Autodesk Inventor part; units mm, degrees
ref_plane "YZ Plane" through (0, 0, 0) normal (1, 0, 0) x (0, 1, 0)
ref_plane "XZ Plane" through (0, 0, 0) normal (0, 1, 0) x (-1, 0, 0)
ref_plane "XY Plane" through (0, 0, 0) normal (0, 0, 1) x (1, 0, 0)
sketch "Sketch1" plane through (0, 0, 0) normal (0, 1, 0) x (-1, 0, 0)
  circle A0 centre (0, 0) radius 2.3241
  line L0 (0, 0) -> (0, -38.1)
  circle A1 centre (0, -38.1) radius 2.3241
  line L1 (0, 0) -> (0, -38.1) construction
  line L2 (-6.35, 0) -> (-6.35, -38.1)
  line L3 (6.35, -38.1) -> (6.35, 0)
  arc A2 (6.35, 0) -> (-6.35, 0) centre (0, 0) ccw
  arc A3 (-6.35, -38.1) -> (6.35, -38.1) centre (0, -38.1) ccw
  line L4 (0, -38.1) -> (-15.9411, -38.1) construction
  line L5 (0, -31.75) -> (-15.9411, -31.75)
  line L6 (-15.9411, -44.45) -> (0, -44.45)
  arc A4 (0, -44.45) -> (0, -31.75) centre (0, -38.1) ccw
  arc A5 (-15.9411, -31.75) -> (-15.9411, -44.45) centre (-15.9411, -38.1) ccw
  line L7 (-5.9094, 2.3241) -> (-21.799, -35.6488)
  point P0 (0, -19.05)
  point P1 (-7.9706, -38.1)
  dimension "d0" = 4.6482
  dimension "d1" = 38.1
  dimension "d2" = 4.6482
  dimension "d3" = 12.7
extrude "Extrusion1" add sketch "Sketch1" along normal blind 1.5875
sketch "Sketch2" plane through (0, 1.5875, 0) normal (0, 1, 0) x (1, 0, 0)
  circle A0 centre (0, 38.1) radius 2.3241
  line L0 (0, 38.1) -> (0, 31.75)
  line L1 (0, 31.75) -> (0, 92.71) construction
  line L2 (6.35, 38.1) -> (6.35, 86.36)
  line L3 (-6.35, 86.36) -> (-6.35, 38.1)
  arc A1 (-6.35, 38.1) -> (6.35, 38.1) centre (0, 38.1) ccw
  arc A2 (6.35, 86.36) -> (-6.35, 86.36) centre (0, 86.36) ccw
  line L4 (-6.35, 86.36) -> (57.15, 86.36) construction
  line L5 (0, 80.01) -> (50.8, 80.01)
  line L6 (50.8, 92.71) -> (0, 92.71)
  arc A3 (0, 92.71) -> (0, 80.01) centre (0, 86.36) ccw
  arc A4 (50.8, 80.01) -> (50.8, 92.71) centre (50.8, 86.36) ccw
  line L7 (-6.35, 38.1) -> (-6.35, 0)
  arc A5 (-6.35, 0) -> (5.9094, -2.3241) centre (0, 0) ccw
  line L8 (5.9094, -2.3241) -> (21.799, 35.6488)
  arc A6 (21.799, 35.6488) -> (15.9411, 44.45) centre (15.9411, 38.1) ccw
  line L9 (15.9411, 44.45) -> (0, 44.45)
  arc A7 (0, 44.45) -> (-6.35, 38.1) centre (0, 38.1) ccw
  circle A8 centre (0, 0) radius 2.3241
  circle A9 centre (0, 38.1) radius 2.3241
  line L10 (21.799, 35.6488) -> (55.9369, 82.6271)
  point P0 (0, 62.23)
  point P1 (25.4, 86.36)
  point P2 (0, 92.71)
  point P3 (6.35, 44.45)
  dimension "d6" = 6.35
  dimension "d7" = 60.96
  dimension "d10" = 63.5
extrude "Extrusion2" add sketch "Sketch2" against normal blind 1.5875 contours A1 A7 L9 L2 | L9 A7 L3 A3 L5 L2 | L2 L5 A4 L10 A6 L9 | L5 A3 A2 L2 | L2 A2 L6 A4 L5
sketch "Sketch3" plane through (0, 1.5875, 0) normal (0, 1, 0) x (1, 0, 0)
  arc A0 (55.9369, 82.6271) -> (50.8, 92.71) centre (50.8, 86.36) ccw
  line L0 (5.9094, -2.3241) -> (21.799, 35.6488)
  arc A1 (55.9369, 82.6271) -> (5.9094, -2.3241) centre (174.4039, -44.3439) ccw
  line L1 (21.799, 35.6488) -> (55.9369, 82.6271)
  point P0 (0, 0)
extrude "Extrusion3" cut sketch "Sketch3" against normal blind 1.5875
sketch "Sketch4" plane through (0, 1.5875, 0) normal (0, 1, 0) x (1, 0, 0)
  line L0 (0, 92.71) -> (50.8, 92.71)
  line L1 (-6.35, 86.36) -> (-6.35, 0)
  arc A0 (30.6634, 92.71) -> (-6.35, 43.18) centre (81.4918, 16.1314) ccw
  arc A1 (55.9369, 82.6271) -> (5.9094, -2.3241) centre (174.4039, -44.3439) ccw
  arc A2 (55.9369, 82.6271) -> (50.8, 92.71) centre (50.8, 86.36) ccw
  line L2 (50.8, 92.71) -> (0, 92.71)
  arc A3 (0, 92.71) -> (-6.35, 86.36) centre (0, 86.36) ccw
  line L3 (-6.35, 86.36) -> (-6.35, 0)
  arc A4 (-6.35, 0) -> (5.9094, -2.3241) centre (0, 0) ccw
  circle A5 centre (0, 0) radius 2.3241
  circle A6 centre (0, 38.1) radius 2.3241
extrude "Extrusion4" cut sketch "Sketch4" against normal blind 1.5875 contours L0 A0 L1 A3
sketch "Sketch5" plane through (0, 1.5875, 0) normal (0, 1, 0) x (1, 0, 0)
  point P0 (0, 0)
sketch "Sketch6" plane through (0, 1.5875, 0) normal (0, 1, 0) x (1, 0, 0)
  circle A0 centre (0, 38.1) radius 2.3241
  line L0 (0, 38.1) -> (0, 50.8)
  circle A1 centre (0, 50.8) radius 2.3241
  point P0 (0, 0)
  dimension "d15" = 12.7
  dimension "d16" = 4.6482
extrude "Extrusion5" cut sketch "Sketch6" against normal blind 1.5875 contours A1
sketch "Sketch7" plane through (0, 1.5875, 0) normal (0, 1, 0) x (1, 0, 0)
  circle A0 centre (0, 50.8) radius 2.3241
  circle A1 centre (0, 38.1) radius 2.3241
  arc A2 (6.2992, 38.1) -> (-6.2992, 38.1) centre (0, 38.1) ccw
  circle A3 centre (0, 38.1) radius 2.3241
  line L0 (0, 50.8) -> (0, 88.9)
  arc A4 (35.4436, 84.1127) -> (5.3749, 48.0302) centre (101.5031, -1.5067) ccw
  arc A5 (31.75, 88.9) -> (0, 50.8) centre (101.5031, -1.5067) ccw
  arc A6 (31.75, 88.9) -> (0, 50.8) centre (101.5031, -1.5067) ccw construction
  arc A7 (28.0564, 93.6873) -> (-5.3749, 53.5698) centre (101.5031, -1.5067) ccw
  line L1 (0, 88.9) -> (31.75, 88.9)
  arc A8 (35.4436, 84.1127) -> (28.0564, 93.6873) centre (31.75, 88.9) ccw
  line L2 (0, 50.8) -> (6.2992, 50.8)
  circle A9 centre (0, 50.8) radius 2.3241
  arc A10 (6.2992, 50.8) -> (-6.2992, 50.8) centre (0, 50.8) ccw
  line L3 (-6.2992, 50.8) -> (0, 50.8)
  arc A11 (-5.3749, 53.5698) -> (5.3749, 48.0302) centre (0, 50.8) ccw
  line L4 (-6.2992, 38.1) -> (-6.2992, 50.8)
  line L5 (0, 38.1) -> (0, 50.8) construction
  line L6 (6.2992, 50.8) -> (6.2992, 38.1)
  circle A12 centre (0, 38.1) radius 2.3241
  circle A13 centre (31.75, 88.9) radius 2.3241
  point P0 (0, 0)
  point P1 (0, 44.45)
  point P2 (-4.5326, 55.1744)
  point P3 (6.2992, 49.7843)
  point P4 (0, 57.0992)
  point P5 (2.3241, 50.8)
  point P6 (0, 53.1241)
  dimension "d19" = 4.6482
  dimension "d40" = 4.6482
extrude "Extrusion6" add sketch "Sketch7" against normal blind 1.5875 contours L2 L6 A4 A11 L3 A0 | L3 A11 A7 A10 L0 A0 | A10 A5 A13 L1 A7 A8 A4 L6 | A10 L0 A7 L1 A13 A5 | A11 A4 L6 A2 L4 L3 | L3 A10 A7 A11 | A10 A7 L0 | A13 L1 A5 | A5 L1 A13
sketch "Sketch8" plane through (0, 1.5875, 0) normal (0, 1, 0) x (1, 0, 0)
  circle A0 centre (0, 50.8) radius 2.3241
  circle A1 centre (0, 38.1) radius 2.3241
  circle A2 centre (0, 0) radius 2.3241
  arc A3 (36.4452, 92.71) -> (28.0564, 93.6873) centre (31.75, 88.9) ccw
  arc A4 (28.0564, 93.6873) -> (-4.5326, 55.1744) centre (101.5031, -1.5067) ccw
  arc A5 (-4.5326, 55.1744) -> (-6.2992, 50.8) centre (0, 50.8) ccw
  line L0 (-6.2992, 50.8) -> (-6.2992, 43.3444)
  arc A6 (-6.2992, 43.3444) -> (-6.35, 43.18) centre (81.4918, 16.1314) ccw
  line L1 (-6.35, 43.18) -> (-6.35, 0)
  arc A7 (-6.35, 0) -> (5.9094, -2.3241) centre (0, 0) ccw
  arc A8 (55.9369, 82.6271) -> (5.9094, -2.3241) centre (174.4039, -44.3439) ccw
  arc A9 (55.9369, 82.6271) -> (50.8, 92.71) centre (50.8, 86.36) ccw
  line L2 (50.8, 92.71) -> (36.4452, 92.71)
  arc A10 (55.9369, 82.6271) -> (50.8, 92.71) centre (50.8, 86.36) ccw
  line L3 (51.4711, 92.6744) -> (32.4545, 94.9054)
extrude "Extrusion7" add sketch "Sketch8" against normal blind 1.5875 contours A3 L3 A9 L2
sketch "Sketch11" plane through (0, 1.5875, 0) normal (0, 1, 0) x (1, 0, 0)
  arc A0 (55.9369, 82.6271) -> (5.9094, -2.3241) centre (174.4039, -44.3439) ccw
  line L0 (38.9499, 64.3219) -> (56.735, 60.5286)
  line L1 (56.735, 60.5286) -> (50.1783, 76.9989)
  circle A1 centre (0, 50.8) radius 2.3241
  circle A2 centre (0, 38.1) radius 2.3241
  circle A3 centre (0, 0) radius 2.3241
  arc A4 (32.4545, 94.9054) -> (28.0564, 93.6873) centre (31.75, 88.9) ccw
  arc A5 (28.0564, 93.6873) -> (-4.5326, 55.1744) centre (101.5031, -1.5067) ccw
  arc A6 (-4.5326, 55.1744) -> (-6.2992, 50.8) centre (0, 50.8) ccw
  line L2 (-6.2992, 50.8) -> (-6.2992, 43.3444)
  arc A7 (-6.2992, 43.3444) -> (-6.35, 43.18) centre (81.4918, 16.1314) ccw
  line L3 (-6.35, 43.18) -> (-6.35, 0)
  arc A8 (-6.35, 0) -> (5.9094, -2.3241) centre (0, 0) ccw
  arc A9 (55.9369, 82.6271) -> (5.9094, -2.3241) centre (174.4039, -44.3439) ccw
  arc A10 (55.9369, 82.6271) -> (51.4711, 92.6744) centre (50.8, 86.36) ccw
  line L4 (51.4711, 92.6744) -> (32.4545, 94.9054)
extrude "Extrusion10" add sketch "Sketch11" against normal blind 1.5875 contours L1 L0 A0
fillet "Fillet4" radius 12.7 2 edges at (50.1783, 0.7937, -76.9989) (38.9499, 0.7937, -64.3219)
fillet "Fillet5" radius 1.5875 1 edges at (56.735, 0.7937, -60.5286)
extrude "Extrusion11" cut sketch "Sketch7" against normal blind 1.5875 contours A13 L1 A5 | A5 L1 A13
fillet "Fillet6" radius 127 1 edges at (-4.5326, 0.7937, -55.1744)
properties part number "Lady Brown Tabs"
CAD build for the part. Positions are in the model's coordinates, mm. A direction names the side the tool comes from. Give positions to 0.01 mm unless a question says otherwise; leave off trailing zeros. Loops run counter-clockwise (first coordinate to the right, second up) from the corner with the lowest first, then second, coordinate; pieces in that order, holes last. Notation, with made-up numbers: M -0.5,-36 L 47.5,-36 A16 cw 47.5,-7 Z; hole C -27.5,-1.75 d4. An arc over 180 degrees is marked long. Answer in a Markdown table with one row per item. Add a question column.
Item 1: Mould opens along Z. For faces 1 (the face through (33.967, 0.805, -89.598)), 2 (the face through (18, 1.588, -56)), 3 (the face through (-1.06, 0.78, 6.26)) say: +Z half, -Z half, draft (parallel to the pull), parting line (faces both ways), or undercut.
Item 2: Band-saw the part on D-D on x = 19. Give the cut face in (y, z), then the cut area to 3 significant figures.
Item 3: Probe probe 1 along Z at (x, y) = (0, 1.15); probe 2 along X at (y, z) = (1.2, 0); probe 3 along Z at (x, y) = (-1, 0.1). List the from-to ranges inside material, lowest first.
Item 4: Band-saw the part on A-A on x = 0. Give the cut face in (y, z).
Item 5: Band-saw the part on B-B on z = -37. Give the cut face in (x, y), then the cut area to 3 significant figures.
Item 6: Band-saw the part on C-C on z = -88.9. Give the cut face in (x, y), then the cut area to 3 significant figures.
Item 7: Tool access for faces 4 (the face through (0.303, 0.783, -40.404)), 5 (the face through (54.49, 0.8, -66.17)): list every direction of +Z, -Z, +X, -X, +Y, -Y with a clear straight run to the whole face (end or side of a thin tool).
Reply:
| question | item | result |
|---|---|---|
| 1 | face 1 | undercut |
| 1 | face 2 | draft |
| 1 | face 3 | +Z half |
| 2 | outline | M 0,-85.96 L 1.59,-85.96 L 1.59,-33.15 L 0,-33.15 Z |
| 2 | area | 83.8 mm^2 |
| 3 | probe 1 | z = -62.94 to -53.12, -48.48 to -40.42, -35.78 to -2.32, 2.32 to 6.35 |
| 3 | probe 2 | x = -6.35 to -2.32, 2.32 to 6.51 |
| 3 | probe 3 | z = -61.34 to -52.9, -48.7 to -40.2, -36 to -2.1, 2.1 to 6.27 |
| 4 | outline | M 0,-62.94 L 1.59,-62.94 L 1.59,-53.12 L 0,-53.12 Z; M 0,-48.48 L 1.59,-48.48 L 1.59,-40.42 L 0,-40.42 Z; M 0,-35.78 L 1.59,-35.78 L 1.59,-2.32 L 0,-2.32 Z; M 0,2.32 L 1.59,2.32 L 1.59,6.35 L 0,6.35 Z |
| 5 | outline | M -6.35,0 L -2.05,0 L -2.05,1.59 L -6.35,1.59 Z; M 2.05,0 L 20.98,0 L 20.98,1.59 L 2.05,1.59 Z |
| 5 | area | 36.9 mm^2 |
| 6 | outline | M 22.24,0 L 29.43,0 L 29.43,1.59 L 22.24,1.59 Z; M 34.07,0 L 56.62,0 L 56.62,1.59 L 34.07,1.59 Z |
| 6 | area | 47.2 mm^2 |
| 7 | face 4 | +Y, -Y |
| 7 | face 5 | +X, +Y, -Y |
